Autodesk Inventor part; units mm, degrees
ref_plane "Pracovní rovina1" through (0, 0, -30) normal (0, 0, -1) x (-1, 0, 0)
ref_plane "YZ Plane" through (0, 0, 0) normal (1, 0, 0) x (0, 1, 0)
ref_plane "XZ Plane" through (0, 0, 0) normal (0, 1, 0) x (-1, 0, 0)
sketch "Náčrt1" plane through (0, 0, 0) normal (0, 1, 0) x (-1, 0, 0)
  arc A0 (-19, 0) -> (19, 0) centre (0, 0) ccw
  arc A1 (-27.4129, -12.1875) -> (27.4129, -12.1875) centre (0, 0) ccw
  line L0 (56, 0) -> (56, -11)
  line L1 (56, -11) -> (29.2404, -11)
  line L2 (-51, 0) -> (-51, -41)
  line L3 (-51, -41) -> (-40, -41)
  line L4 (-40, -41) -> (-40, -13)
  line L5 (-38, -11) -> (-29.2404, -11)
  arc A2 (29.2404, -11) -> (27.4129, -12.1875) centre (29.2404, -13) ccw
  arc A3 (-27.4129, -12.1875) -> (-29.2404, -11) centre (-29.2404, -13) ccw
  arc A4 (-38, -11) -> (-40, -13) centre (-38, -13) ccw
  line L6 (56, 0) -> (19, 0)
  line L7 (-19, 0) -> (-51, 0)
  point P0 (27.9106, -11)
  point P1 (-27.9106, -11)
  dimension "d0" = 19
  dimension "d1" = 30
  dimension "d3" = 107
  dimension "d4" = 51
  dimension "d5" = 11
  dimension "d6" = 41
  dimension "d7" = 11
  dimension "d8" = 2
  dimension "d9" = 2
  dimension "d10" = 2
  dimension "d16" = 96
  dimension "d17" = 56
extrude "Vysunutí1" add sketch "Náčrt1" against normal blind 48
fillet "Zaoblení1" radius 13 1 edges at (-56, 0, -5.5)
fillet "Zaoblení2" radius 13 1 edges at (-56, -48, -5.5)
fillet "Zaoblení3" radius 6 2 edges at (45.5, -48, -41) (45.5, 0, -41)
sketch "Náčrt2" plane through (-29.2404, -48, -11) normal (0, 0, -1) x (-1, 0, 0)
  line L0 (-56.6532, 0) -> (-1.8275, 0)
  circle A0 centre (13.7596, 13) radius 5
  circle A1 centre (13.7596, 35) radius 5
  point P0 (-29.2404, 48)
  dimension "d26" = 10
  dimension "d27" = 10
  dimension "d28" = 35
  dimension "d29" = 13
  dimension "d30" = 38.3139
  dimension "d31" = 20.2968
extrude "Vysunutí2" cut sketch "Náčrt2" against normal blind 11
ref_plane "Pracovní rovina1" through (0, 0, -30) normal (0, 0, -1) x (-1, 0, 0)
sketch "Náčrt3" plane through (0, 0, -30) normal (0, 0, -1) x (-1, 0, 0)
  circle A0 centre (0, -24) radius 2.5
  point P0 (0, 0)
  dimension "d34" = 5
hole "Díra1" at (0, -24, -30) direction (0, 0, 1) diameter 4.9784 end through all
sketch "Náčrt4" plane through (51, -48, 0) normal (1, 0, 0) x (0, 0, -1)
  line L0 (0, 48) -> (0, 0)
  line L1 (0, 48) -> (35, 48)
  arc A0 (25, 30.5) -> (25, 17.5) centre (25, 24) ccw
  line L2 (25, 30.5) -> (41, 30.5)
  line L3 (25, 17.5) -> (41, 17.5)
  line L4 (41, 17.5) -> (41, 30.5)
  dimension "d45" = 13
  dimension "d46" = 24
  dimension "d47" = 25
  dimension "d48" = 41
extrude "Vysunutí3" cut sketch "Náčrt4" against normal blind 11
properties part number "3"
CAD build for the part. Positions are in the model's coordinates, mm. A direction names the side the tool comes from. Round coordinates to 2 decimals unless told otherwise and drop trailing zeros. Write each loop counter-clockwise with the first axis right and the second up, starting at its lowest first coordinate (ties: lowest second). Pieces come first, ordered by that corner, then holes.
Item 1: Tool access for faces 4 (the flat face through (-43, -24, -11)), 5 (the cylindrical face through (39.4, -23.66, -11.57)), 6 (the flat face through (46, -17.5, -33)), 7 (the cylindrical face through (-0.109, -26.487, -24.34)), 8 (the flat face through (-38, -24, 0)): list every direction of +Z, -Z, +X, -X, +Y, -Y with a clear straight run to the whole face (end or side of a thin tool).
Filled in:
face 4: -Z, -X, +Y, -Y
face 5: -Z, +Y, -Y
face 6: -Z, +X
face 7: +Z, -Z
face 8: +Z, +X, -X, +Y, -Y
Item 2: Band-saw the part on D-D on y = -5. Write the cut outline in (x, z).
Filled in:
outline: (-53.25, -11) - (-29.24, -11) arc R2 cw to (-27.41, -12.19) arc R30 ccw to (27.41, -12.19) arc R2 cw to (29.24, -11) - (38, -11) arc R2 cw to (40, -13) - (40, -40.92) - (51, -40.92) - (51, 0) - (19, 0) arc R19 cw to (-19, 0) - (-53.25, 0) - close
Item 3: Mould opens along X. For faces 1 (the cylindrical face through (0, -18, -30)), 2 (the cylindrical face through (45.423, -1.711, -39.196)), 3 (the flat face through (-56, -24, -5)) say: released by +X, released by -X, zero draft, split by the parting line, or undercut.
Filled in:
face 1: undercut
face 2: zero draft
face 3: released by -X
Item 4: Drop flat-ended pins along their axis: pin 1 Ø2.5 at (x, y) = (32, -15) entering from -Z; pin 2 Ø1 at (x, y) = (-23, -20.5) entering from -Z; pin 3 Ø12 at (y, z) = (-7, -29) entering from -X; pin 4 Ø6 at (x, y) = (-43, -13) entering from -Z. Give the stop position or say it passes through.
Filled in:
pin 1: stops at z = -11
pin 2: stops at z = -19.84
pin 3: stops at x = -19.26
pin 4: passes through
Item 5: Band-saw the part on A-A on z = -24. Write the cut outline in (x, y).
Filled in:
outline: (-18, -48) - (18, -48) - (18, 0) - (-18, 0) - close; (40, -48) - (51, -48) - (51, -30.42) - (40, -30.42) - close; (40, -17.58) - (51, -17.58) - (51, 0) - (40, 0) - close; hole circle Ø4.98 at (0, -24)
Item 6: Drill centre lines: L1, parallel to Y at x = -43, z = -7.5; L2, parallel to Y at x = 0, z = -24; L3, parallel to X at y = -11.5, z = -8.5. Where is each one in solid material? Low to high.
Filled in:
L1: y = -48 to -40, -30 to -18, -8 to 0
L2: y = -48 to -26.49, -21.51 to 0
L3: x = -55.91 to -47.77, -38.23 to -16.99, 16.99 to 51
Item 7: Band-saw the part on B-B on z = -3. Write the cut outline in (x, y).
Filled in:
outline: (-56, -35) arc R13 ccw to (-43, -48) - (-18.76, -48) - (-18.76, 0) - (-43, 0) arc R13 ccw to (-56, -13) - close; (18.76, -48) - (51, -48) - (51, 0) - (18.76, 0) - close; hole circle Ø10 at (-43, -35); hole circle Ø10 at (-43, -13)
Item 8: Band-saw the part on C-C on y = -32.5. Write the cut outline in (x, z).
Filled in:
outline: (-56, -11) - (-47.33, -11) - (-47.33, 0) - (-56, 0) - close; (-38.67, -11) - (-29.24, -11) arc R2 cw to (-27.41, -12.19) arc R30 ccw to (27.41, -12.19) arc R2 cw to (29.24, -11) - (38, -11) arc R2 cw to (40, -13) - (40, -41) - (51, -41) - (51, 0) - (19, 0) arc R19 cw to (-19, 0) - (-38.67, 0) - close
